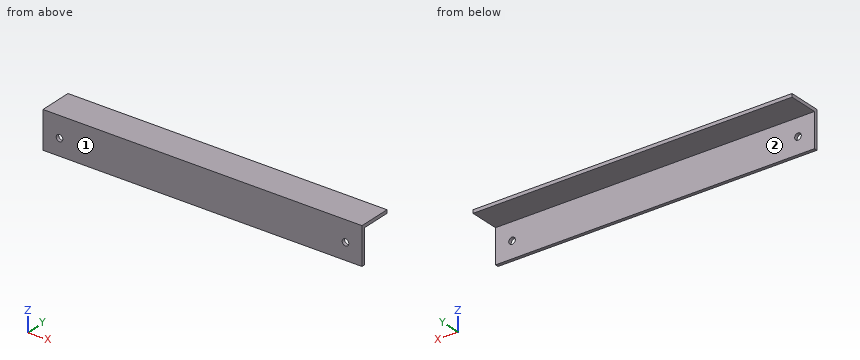
from build123d import *

# Parameters (mm, degrees)
THICKEN1_OUTLINE_W   = 193
THICKEN1_OUTLINE_H   = 22.5
THICKEN1_OUTLINE_R   = 2
THICKEN1_DEPTH       = 2
THICKEN1_START       = 2
THICKEN1_2_OUTLINE_W = 193
THICKEN1_2_OUTLINE_H = 2
THICKEN1_2_DEPTH     = 18


# Read off the part's stored shape, not the designer's step: Thicken1
with BuildPart() as part:
    # Thicken1 outline → Thicken1 (new body)
    with BuildSketch(Plane(origin=(0, 0, 0), x_dir=(1, 0, 0), z_dir=(0, 1, 0))):
        with Locations((96.5, 11.25)):
            Rectangle(THICKEN1_OUTLINE_W, THICKEN1_OUTLINE_H)
        with Locations((10, 12.5)):
            Circle(THICKEN1_OUTLINE_R, mode=Mode.SUBTRACT)
        with Locations((183, 12.5)):
            Circle(THICKEN1_OUTLINE_R, mode=Mode.SUBTRACT)
    extrude(amount=THICKEN1_DEPTH)

    # Thicken1 2 outline → Thicken1 2 (add)
    with BuildSketch(Plane(origin=(0, 0, 0), x_dir=(1, 0, 0), z_dir=(0, 1, 0)).offset(THICKEN1_START)):
        with Locations((96.5, 1)):
            Rectangle(THICKEN1_2_OUTLINE_W, THICKEN1_2_OUTLINE_H)
    extrude(amount=THICKEN1_2_DEPTH)


solid = part.part
Design review of the part built by this model. Coordinates are the model's own, in mm. Face numbers are marked on the shaded views. A direction names the side the tool comes from. Round coordinates to 2 decimals unless told otherwise and drop trailing zeros. Write each loop counter-clockwise with the first axis right and the second up, starting at its lowest first coordinate (ties: lowest second). Pieces come first, ordered by that corner, then holes. Notation, with made-up numbers: (9, -16) - (18, -16) arc R24 cw to (18, -4) - close; hole circle Ø9 at (21, -25.5). An arc over 180 degrees is marked (long way). Use a Markdown table: item, result. Add a question column.
1. We need section D-D (x = 141). State the section outline as (y, z) points, then the cut area to 3 significant figures.
2. For the marked faces 1 and 2, list the 3-axis set-ups (+Z, -Z, +X, -X, +Y, -Y) from which the entire face can be reached by the end or side of a thin tool; tool diameter is ignored.
3. Wall thickness on probe 1 along X at (y, z) = (0.7, -12.5); probe 2 along Z at (x, y) = (183, 0.55); probe 3 along Y at (x, z) = (57.5, -3.75): over which ranges is each line inside the solid? List them lowest first.
4. We need section A-A (z = -12.5). State the section outline as (x, y) points, then the cut area to 3 significant figures.
5. We need section C-C (y = 7.25). State the section outline as (x, z) points.
6. Clearance check with flat-ended pins moving along their axes: pin 1 (1 mm diameter, centred on x = 28, y = 11.5, fed in from -Z); pin 2 (3 mm diameter, centred on x = 183, z = -12.5, fed in from -Y); pin 3 (1 mm diameter, centred on x = 24, z = -15, fed in from +Y). State where each tip first meets the part, or that it passes through.
7. We need section B-B (x = 183). State the section outline as (y, z) points.
Output:
| question | item | result |
|---|---|---|
| 1 | outline | (0, -22.5) - (2, -22.5) - (2, -2) - (20, -2) - (20, 0) - (0, 0) - close |
| 1 | area | 81.0 mm2 |
| 2 | face 1 | +Z, -Z, +X, -X, -Y |
| 2 | face 2 | -Z, +X, -X, +Y |
| 3 | probe 1 | x = 0 to 8, 12 to 181, 185 to 193 |
| 3 | probe 2 | z = -22.5 to -14.5, -10.5 to 0 |
| 3 | probe 3 | y = 0 to 2 |
| 4 | outline | (0, 0) - (8, 0) - (8, 2) - (0, 2) - close; (12, 0) - (181, 0) - (181, 2) - (12, 2) - close; (185, 0) - (193, 0) - (193, 2) - (185, 2) - close |
| 4 | area | 370 mm2 |
| 5 | outline | (0, -2) - (193, -2) - (193, 0) - (0, 0) - close |
| 6 | pin 1 | stops at z = -2 |
| 6 | pin 2 | passes through |
| 6 | pin 3 | stops at y = 2 |
| 7 | outline | (0, -22.5) - (2, -22.5) - (2, -14.5) - (0, -14.5) - close; (0, -10.5) - (2, -10.5) - (2, -2) - (20, -2) - (20, 0) - (0, 0) - close |
